```python
from build123d import *

# Parameters (mm, degrees)
F0_R      = 7.5
F1_DEPTH  = 150
F2_R      = 6
F3_DEPTH  = 300
F4_R      = 7.5
F5_DEPTH  = 80
F6_R      = 6
F7_DEPTH  = 80
F8_R      = 7.5
F9_DEPTH  = 150
F10_R     = 6
F11_DEPTH = 300
F12_R     = 6
F13_DEPTH = 300


with BuildPart() as f1:
    # F0 (on Top) → F1 (new body)
    with BuildSketch(Plane.XY):
        Circle(F0_R)
    extrude(amount=F1_DEPTH)

    # F2 (on face) → F3 (cut)
    with BuildSketch(Plane.XY):
        Circle(F2_R)
    extrude(amount=-F3_DEPTH, mode=Mode.SUBTRACT)

    # F4 (on Right) → F5 (join)
    with BuildSketch(Plane.YZ):
        with Locations((0, 7.5)):
            Circle(F4_R)
    extrude(amount=F5_DEPTH)

    # F6 (on face) → F7 (cut)
    with BuildSketch(Plane.YZ.offset(80)):
        with Locations((0, 7.5)):
            Circle(F6_R)
    extrude(amount=-F7_DEPTH, mode=Mode.SUBTRACT)

    # F8 (on Top) → F9 (join)
    with BuildSketch(Plane.XY):
        with Locations((80, 0)):
            Circle(F8_R)
    extrude(amount=F9_DEPTH)

    # F10 (on face) → F11 (cut)
    with BuildSketch(Plane.XY.offset(150)):
        with Locations((80, 0)):
            Circle(F10_R)
    extrude(amount=-F11_DEPTH, mode=Mode.SUBTRACT)

    # F12 (on Top) → F13 (cut)
    with BuildSketch(Plane.XY):
        Circle(F12_R)
    extrude(amount=F13_DEPTH, mode=Mode.SUBTRACT)


solid = f1.part
```
The model under review builds one solid part; all positions refer to its coordinate system, in mm. A direction names the side the tool comes from. Round coordinates to 2 decimals unless told otherwise and drop trailing zeros. Order: outer loops, then holes, each group sorted by start corner. A loop starts at its lowest first (then second) coordinate and runs counter-clockwise, first axis right, second up. Notation, with made-up numbers: (28, 14.5) -> (77, 14.5) arc R15 cw to (77, 31.5) -> close; hole circle Ø10 at (-39.75, 67). An arc over 180 degrees is marked (long way). One line per item, written item: value. Start each with the question number.
Q1. Take a section at D-D (x = 56). Write out the cut boundary in (y, z), and give its area (3 significant figures).
Q2. Wall thickness on line 1 (Z direction, x = 49, y = -0.5); line 2 (X direction, y = -5.5, z = 101.5); line 3 (X direction, y = 4, z = 142.5): over which ranges is each line inside the solid? List them lowest first.
Q3. Mouldability with a two-part tool opening along X and no side actions: class faces 3 (the face through (82, 6, 150)), 4 (the face through (-7.493, 0.33, 73.95)) as released by +X, released by -X, zero draft, split by the parting line, or undercut.
Q4. Take a section at B-B (y = -2.75). Write out the cut boundary in (x, z), and give its area (3 significant figures).
Q5. Take a section at A-A (z = 81.5). Write out the cut boundary in (x, y).
Q6. Take a section at C-C (z = 7.5). Write out the cut boundary in (x, y).
Q7. Clearance check with flat-ended pins moving along their axes: pin 1 Ø3 at (y, z) = (2.5, 102) entering from +X; pin 2 Ø4 at (x, y) = (50, 4.5) entering from +Z; pin 3 Ø2 at (x, y) = (42, 5) entering from +Z; pin 4 Ø7 at (x, y) = (80, 0) entering from -Z. State where each tip first meets the part, or that it passes through.
Q8. Machinability: for faces 1 (the face through (-6, 0, 74)), 2 (the face through (39.44, 6.93, 4.63)), which of the approach directions +Z, -Z, +X, -X, +Y, -Y give a long, thin tool a straight path to every point of the face, cutting with its end or side? Answer none if there is none.
Reported:
1. outline: circle Ø15 at (0, 7.5); hole circle Ø12 at (0, 7.5)
1. area: 63.6 mm2
2. line 1: z = 0.02 to 1.52, 13.48 to 14.98
2. line 2: x = -5.1 to -2.4, 2.4 to 5.1, 74.9 to 77.6, 82.4 to 85.1
2. line 3: x = -6.34 to -4.47, 4.47 to 6.34, 73.66 to 75.53, 84.47 to 86.34
3. face 3: zero draft
3. face 4: undercut
4. outline: (-6.98, 0) -> (-5.33, 0) -> (-5.33, 150) -> (-6.98, 150) -> close; (5.33, 0) -> (6.98, 0) -> (6.98, 0.52) -> (73.02, 0.52) -> (73.02, 0) -> (74.67, 0) -> (74.67, 150) -> (73.02, 150) -> (73.02, 14.48) -> (6.98, 14.48) -> (6.98, 150) -> (5.33, 150) -> (5.33, 12.83) -> (73.02, 12.83) -> (73.02, 2.17) -> (5.33, 2.17) -> close; (85.33, 0) -> (86.98, 0) -> (86.98, 150) -> (85.33, 150) -> close
4. area: 1,190 mm2
5. outline: circle Ø15 at (0, 0); circle Ø15 at (80, 0); hole circle Ø12 at (0, 0); hole circle Ø12 at (80, 0)
6. outline: (0, -7.5) -> (80, -7.5) arc R7.5 ccw to (80, 7.5) -> (0, 7.5) arc R7.5 ccw to start; hole (0, -6) -> (75.5, -6) arc R7.5 cw to (75.5, 6) -> (0, 6) arc R6 ccw to start; hole circle Ø12 at (80, 0)
7. pin 1: stops at x = 87.43
7. pin 2: stops at z = 14.57
7. pin 3: stops at z = 13.84
7. pin 4: passes through
8. face 1: +Z, -Z
8. face 2: none
